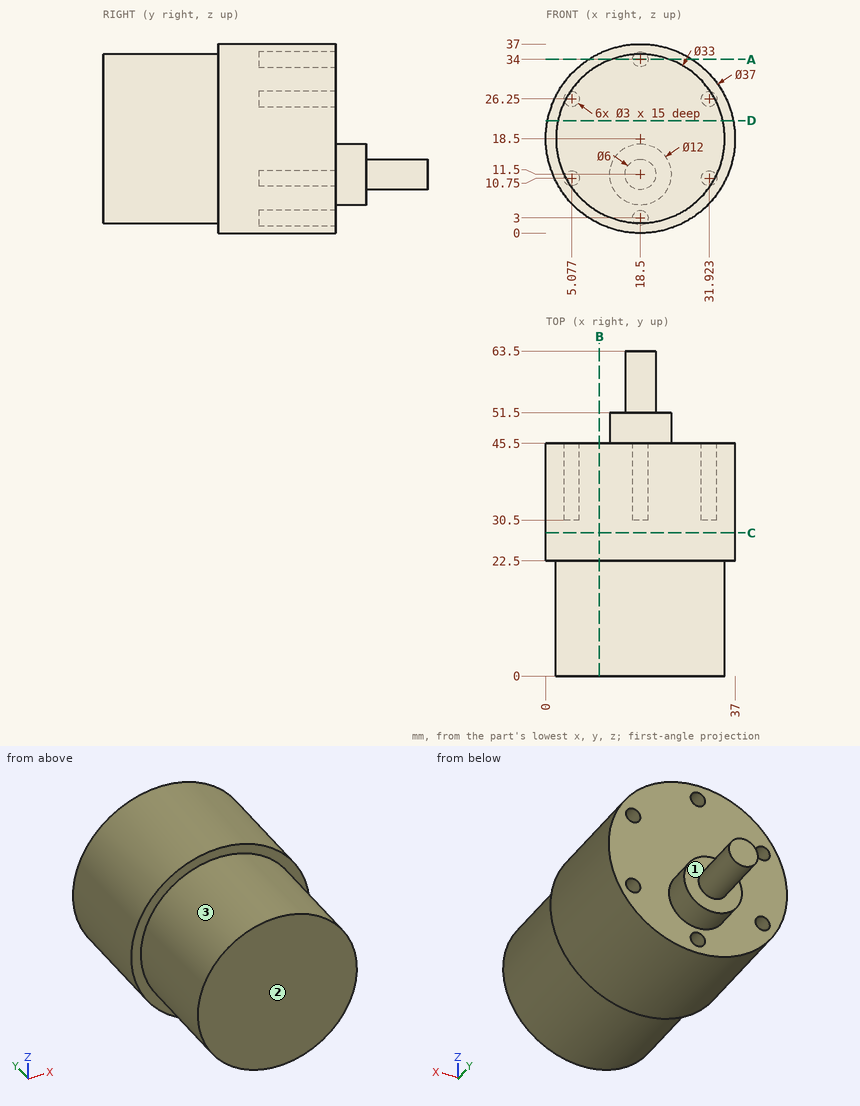
Input: dimensioned drawing with shaded views. Units: mm. Origin: part minimum x, y, z. A direction names the side the tool comes from. Give positions to 0.01 mm unless a question says otherwise; leave off trailing zeros. Write each loop counter-clockwise with the first axis right and the second up, starting at its lowest first coordinate (ties: lowest second). Pieces come first, ordered by that corner, then holes. Notation, with made-up numbers: (-26, 56.25) -> (-5, 56.25) arc R9 ccw to (-5, 62.25) -> close; hole circle Ø6 at (-8, 87.25). An arc over 180 degrees is marked (long way). Answer as a JSON object with one key per item and string values.
1. Contact query for flat-ended pins moving along their axis: pin 1 (8 mm diameter, centred on x = 9.5, y = 34, fed in from -Z); pin 2 (1.5 mm diameter, centred on x = 5, z = 11, fed in from +Y); pin 3 (8 mm diameter, centred on y = 52.5, z = 5, fed in from +X) (1 decimal). Output: stop coordinate, or through.
Ans:
{"pin 1": "stops at z = 0.69", "pin 2": "stops at y = 30.5", "pin 3": "stops at x = 23.9"}
2. Cut plane B-B on x = 10.5. Output: boundary loops of the cut face in (y, z).
Ans:
{"outline": "(0, 4.07) -> (22.5, 4.07) -> (22.5, 1.82) -> (45.5, 1.82) -> (45.5, 35.18) -> (22.5, 35.18) -> (22.5, 32.93) -> (0, 32.93) -> close"}
3. Cut plane A-A on z = 34. Output: boundary loops of the cut face in (x, y).
Ans:
{"outline": "(8.4, 22.5) -> (12.84, 22.5) -> (12.84, 0) -> (24.16, 0) -> (24.16, 22.5) -> (28.6, 22.5) -> (28.6, 45.5) -> (20, 45.5) -> (20, 30.5) -> (17, 30.5) -> (17, 45.5) -> (8.4, 45.5) -> close"}
4. Cut plane D-D on z = 22. Output: boundary loops of the cut face in (x, y) (1 decimal), and give its area (3 significant figures).
Ans:
{"outline": "(0.3, 22.5) -> (2.4, 22.5) -> (2.4, 0) -> (34.6, 0) -> (34.6, 22.5) -> (36.7, 22.5) -> (36.7, 45.5) -> (0.3, 45.5) -> close", "area": "1,560 mm^2"}
5. Ray query, probe 1 along Z at (x, y) = (18, 41) (1 decimal); probe 2 along X at (y, z) = (37, 26) (1 decimal); probe 3 along Y at (x, z) = (19.5, 27). Return the intervals inside material, ascending. Write a range as from..to.
Ans:
{"probe 1": "z = 0..1.6, 4.4..32.6, 35.4..37", "probe 2": "x = 1.6..3.6, 6.6..30.4, 33.4..35.4", "probe 3": "y = 0..45.5"}
6. Cut plane C-C on y = 28. Output: boundary loops of the cut face in (x, z).
Ans:
{"outline": "circle Ø37 at (18.5, 18.5)"}
7. Access query for the marked faces 1, 2 and 3. Directions: +Z, -Z, +X, -X, +Y, -Y. A direction counts if a zero-diameter tool reaches every point of the face in a straight line with its end or side. Return the directions, or none.
Ans:
{"face 1": "+Y", "face 2": "+Z, -Z, +X, -X, -Y", "face 3": "-Y"}
